Can you work these out from the drawing? Everything is in mm from the part's minimum corner. Give positions to 0.01 mm unless a question says otherwise; leave off trailing zeros. Order: outer loops, then holes, each group sorted by start corner. A loop starts at its lowest first (then second) coordinate and runs counter-clockwise, first axis right, second up. Notation, with made-up numbers: (26.25, -36.5) -> (69.25, -36.5) arc R20 ccw to (69.25, -4.5) -> close; hole circle Ø8 at (-37.75, -13.5). An arc over 180 degrees is marked (long way). Answer as CSV lines item,"result". Start each with the question number.
(1) I want a section at A-A (z = 6.5). Please give me the cut outline in (x, y), plus the area to 3 significant figures.
(2) I need wall thicknesses on L1, parallel to X at y = 10.5, z = 1.25 (1 decimal); L2, parallel to X at y = 9.5, z = 6.5; L3, parallel to Y at x = 22, z = 8.5 (1 decimal). Which ranges of each line are inside material? Lowest first, please.
(3) I want a section at C-C (y = 9). Please give me the cut outline in (x, z).
(4) I want a section at B-B (x = 21). Please give me the cut outline in (y, z).
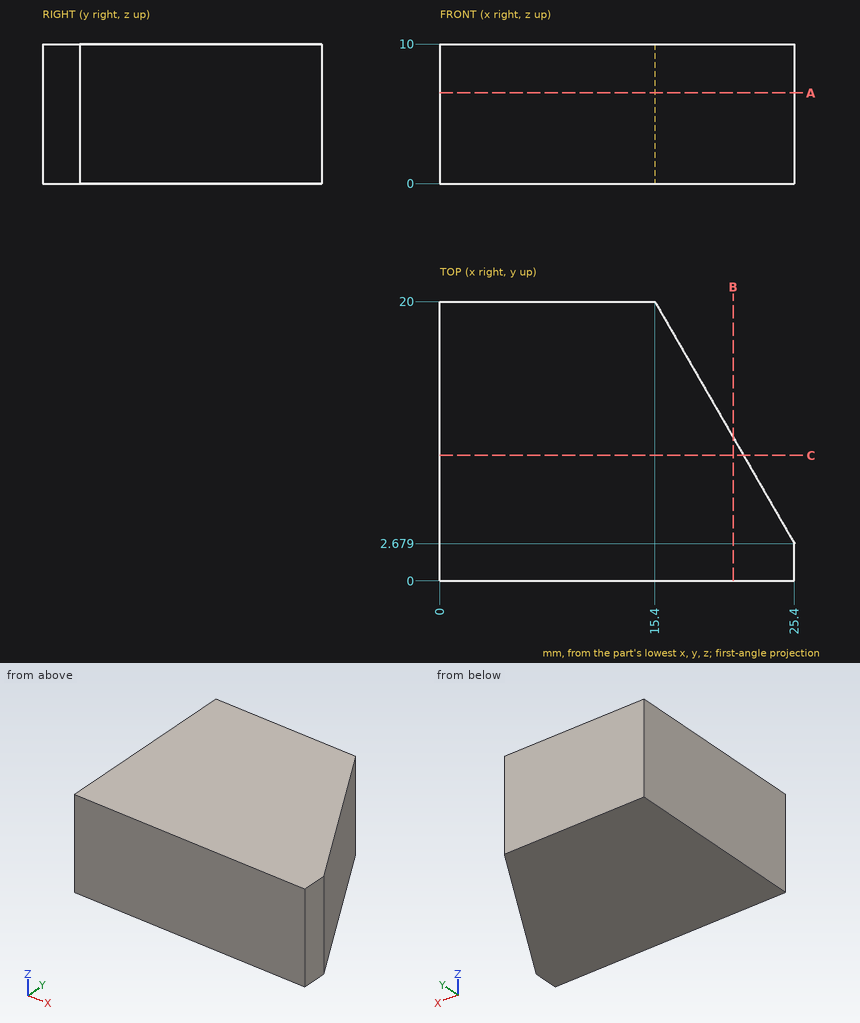
Final values:
1,outline,"(0, 0) -> (25.4, 0) -> (25.4, 2.68) -> (15.4, 20) -> (0, 20) -> close"
1,area,"421 mm²"
2,L1,"0 to 20.9"
2,L2,"0 to 21.46"
2,L3,"0 to 8.6"
3,outline,"(0, 0) -> (21.75, 0) -> (21.75, 10) -> (0, 10) -> close"
4,outline,"(0, 0) -> (10.3, 0) -> (10.3, 10) -> (0, 10) -> close"
